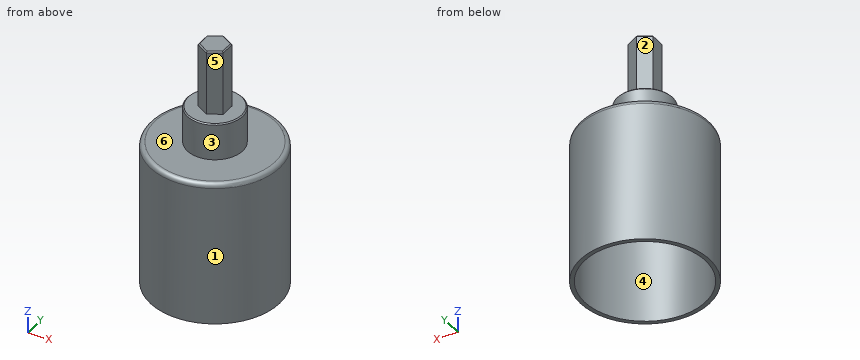
```python
from build123d import *

# Parameters (mm, degrees)
F0_R     = 22.225
F0_R_2   = 9.525
F1_DEPTH = 49.8602
F2_T     = -1.397
F3_R     = 1.5875
F4_DEPTH = 34.925
F5_DEPTH = 12.7
F6_SIZE  = 0.381


with BuildPart() as f1:
    # F0 (on Top) → F1 (new body)
    with BuildSketch(Plane.XY):
        Circle(F0_R)
        Circle(F0_R_2, mode=Mode.SUBTRACT)
        Circle(F0_R_2)
        Polygon((-4.318, 2.4929984624), (0, 4.9859969247), (4.318, 2.4929984624), (4.318, -2.4929984624), (0, -4.9859969247), (-4.318, -2.4929984624), align=None, mode=Mode.SUBTRACT)
        Polygon((4.318, 2.4929984624), (0, 4.9859969247), (-4.318, 2.4929984624), (-4.318, -2.4929984624), (0, -4.9859969247), (4.318, -2.4929984624), align=None)
    extrude(amount=-F1_DEPTH)

    # F2
    f2_openings = [f1.faces().sort_by_distance(p)[0] for p in [
        (0, 0, -49.8602),
    ]]
    offset(amount=F2_T, openings=f2_openings)

    # F3
    f3_edges = [f1.edges().sort_by_distance(p)[0] for p in [
        (-22.225, 0, 0),
    ]]
    fillet(f3_edges, radius=F3_R)

    # F0 (on Top) → F4 (join)
    with BuildSketch(Plane.XY):
        Polygon((4.318, 2.4929984624), (0, 4.9859969247), (-4.318, 2.4929984624), (-4.318, -2.4929984624), (0, -4.9859969247), (4.318, -2.4929984624), align=None)
    extrude(amount=F4_DEPTH)

    # F0 (on Top) → F5 (join)
    with BuildSketch(Plane.XY):
        Circle(F0_R_2)
        Polygon((-4.318, 2.4929984624), (0, 4.9859969247), (4.318, 2.4929984624), (4.318, -2.4929984624), (0, -4.9859969247), (-4.318, -2.4929984624), align=None, mode=Mode.SUBTRACT)
    extrude(amount=F5_DEPTH)

    # F6
    f6_edges = [f1.edges().sort_by_distance(p)[0] for p in [
        (4.318, 0, 34.925),
        (2.159, 3.739498, 34.925),
        (-2.159, 3.739498, 34.925),
        (-4.318, 0, 34.925),
        (-2.159, -3.739498, 34.925),
        (2.159, -3.739498, 34.925),
        (-9.525, 0, 12.7),
    ]]
    chamfer(f6_edges, length=F6_SIZE)


solid = f1.part
```
Part model, mm, in its own coordinate system. Face numbers are marked on the shaded views. A direction names the side the tool comes from. Give positions to 0.01 mm unless a question says otherwise; leave off trailing zeros. Write each loop counter-clockwise with the first axis right and the second up, starting at its lowest first coordinate (ties: lowest second). Pieces come first, ordered by that corner, then holes. Notation, with made-up numbers: (7, 83) -> (11, 83) arc R29 ccw to (11, 110) -> close; hole circle Ø9 at (5, -9.5). An arc over 180 degrees is marked (long way). Put each result on its own line as item: value. Start each with the question number.
Item 1: Cut at B-B (z = -25). List the corners of the cut face in (x, y) (3 decimals).
Item 2: Pull direction X, two halves, no side cores. Call the marked faces 4, 5 and 6: pulls with the +X half, pulls with the -X half, needs draft (parallel to the pull), parting line crosses it, or undercut.
Item 3: Which spindle directions (+Z, -Z, +X, -X, +Y, -Y) get a long thin tool onto all of the face, cutting with end or side? Do the marked faces 1, 2 and 3. Say none if no direction does.
Item 4: Cut at C-C (z = 16). List the corners of the cut face in (x, y), then the cut area to 3 significant figures.
Item 5: Wall check: L1, parallel to Y at x = 0, z = -29 (3 decimals); L2, parallel to Z at x = 7.5, y = 1; L3, parallel to Z at x = -3, y = 14.5. Give the ranges that are in metal, low to high. Write a range as [from, to].
Item 6: Cut at A-A (y = 0). List the corners of the cut face in (x, z) (1 decimal).
Item 7: Pin check, flat tips, straight feed: pin 1 Ø3 at (x, z) = (11, -19.5) entering from -Y; pin 2 Ø5.5 at (y, z) = (1, 20.5) entering from -X; pin 3 Ø8 at (x, y) = (6, -10) entering from -Z. Stop position of each tip, or through.
Answer list:
1. outline: circle Ø44.45 at (0, 0); hole circle Ø41.656 at (0, 0)
2. face 4: undercut
2. face 5: pulls with the +X half
2. face 6: needs draft
3. face 1: +Z, -Z
3. face 2: +Z, -X, +Y
3. face 3: +Z
4. outline: (-4.32, -2.49) -> (0, -4.99) -> (4.32, -2.49) -> (4.32, 2.49) -> (0, 4.99) -> (-4.32, 2.49) -> close
4. area: 64.6 mm2
5. L1: y = [-22.225, -20.828], [20.828, 22.225]
5. L2: z = [-1.4, 12.7]
5. L3: z = [-1.4, 0]
6. outline: (-22.2, -49.9) -> (-20.8, -49.9) -> (-20.8, -1.4) -> (20.8, -1.4) -> (20.8, -49.9) -> (22.2, -49.9) -> (22.2, -1.6) arc R1.6 ccw to (20.6, 0) -> (9.5, 0) -> (9.5, 12.3) -> (9.1, 12.7) -> (4.3, 12.7) -> (4.3, 34.5) -> (3.9, 34.9) -> (-3.9, 34.9) -> (-4.3, 34.5) -> (-4.3, 12.7) -> (-9.1, 12.7) -> (-9.5, 12.3) -> (-9.5, 0) -> (-20.6, 0) arc R1.6 ccw to (-22.2, -1.6) -> close
7. pin 1: stops at y = -20.09
7. pin 2: stops at x = -4.32
7. pin 3: stops at z = -1.4
